The model under review builds one solid part; all positions refer to its coordinate system, in mm. A direction names the side the tool comes from. Round coordinates to 2 decimals unless told otherwise and drop trailing zeros. Write each loop counter-clockwise with the first axis right and the second up, starting at its lowest first coordinate (ties: lowest second). Pieces come first, ordered by that corner, then holes. Notation, with made-up numbers: (35.5, -36.5) - (47.5, -36.5) arc R22 cw to (47.5, -3.5) - close; hole circle Ø11 at (79.5, 10.5). An arc over 180 degrees is marked (long way). Return JSON: item names as keys, results as strings.
from build123d import *

# Parameters (mm, degrees)
BOX002_W          = 1
BOX002_H          = 4.5
BOX002_DEPTH      = 5.75
ARRAY001_COUNT    = 2
BOX001_W          = 2
BOX001_H          = 4.5
BOX001_DEPTH      = 5.5
ARRAY_COUNT       = 2
CYLINDER003_R     = 0.45
CYLINDER003_DEPTH = 2
CYLINDER004_R     = 0.45
CYLINDER004_DEPTH = 2
CYLINDER005_R     = 0.45
CYLINDER005_DEPTH = 2
CYLINDER006_R     = 0.45
CYLINDER006_DEPTH = 2
CYLINDER007_R     = 0.45
CYLINDER007_DEPTH = 2
CYLINDER008_R     = 0.45
CYLINDER008_DEPTH = 2
CYLINDER009_R     = 0.45
CYLINDER009_DEPTH = 2
CYLINDER010_R     = 0.45
CYLINDER010_DEPTH = 2
CYLINDER002_R     = 7
CYLINDER002_DEPTH = 10
CYLINDER001_R     = 11.5
CYLINDER001_DEPTH = 2
BOX_W             = 15
BOX_H             = 15
BOX_DEPTH         = 2
CYLINDER_R        = 13
CYLINDER_DEPTH    = 4.5
CHAMFER_SIZE      = 0.7


with BuildPart() as array001:
    # Box002 → Box002 (new body)
    with BuildSketch(Plane(origin=(8, -2.25, 0.75), x_dir=(1, 0, 0), z_dir=(0, 0, 1))):
        with Locations((0.5, 2.25)):
            Rectangle(BOX002_W, BOX002_H)
    extrude(amount=BOX002_DEPTH)

    # Array001: Array001 ×2 about axis
    array001_axis = Axis((0, 0, 0), (0, 0, 1))


with BuildPart() as array001_1:
    add(array001.part)
    for i in range(1, ARRAY001_COUNT):
        add(array001.part.rotate(array001_axis, i * 360 / ARRAY001_COUNT))


with BuildPart() as array:
    # Box001 → Box001 (new body)
    with BuildSketch(Plane(origin=(7, -2.25, 2), x_dir=(1, 0, 0), z_dir=(0, 0, 1))):
        with Locations((1, 2.25)):
            Rectangle(BOX001_W, BOX001_H)
    extrude(amount=BOX001_DEPTH)

    # Array: Array ×2 about axis
    array_axis = Axis((0, 0, 0), (0, 0, 1))


with BuildPart() as array_1:
    add(array.part)
    for i in range(1, ARRAY_COUNT):
        add(array.part.rotate(array_axis, i * 360 / ARRAY_COUNT))


with BuildPart() as cilindro003:
    # Cylinder003 → Cylinder003 (new body)
    with BuildSketch(Plane(origin=(6, 7.5, 4), x_dir=(1, 0, 0), z_dir=(0, 0, 1))):
        Circle(CYLINDER003_R)
    extrude(amount=CYLINDER003_DEPTH)


with BuildPart() as cilindro004:
    # Cylinder004 → Cylinder004 (new body)
    with BuildSketch(Plane(origin=(-6, 7.5, 4), x_dir=(1, 0, 0), z_dir=(0, 0, 1))):
        Circle(CYLINDER004_R)
    extrude(amount=CYLINDER004_DEPTH)


with BuildPart() as cilindro005:
    # Cylinder005 → Cylinder005 (new body)
    with BuildSketch(Plane(origin=(6, -7.5, 4), x_dir=(1, 0, 0), z_dir=(0, 0, 1))):
        Circle(CYLINDER005_R)
    extrude(amount=CYLINDER005_DEPTH)


with BuildPart() as cilindro006:
    # Cylinder006 → Cylinder006 (new body)
    with BuildSketch(Plane(origin=(-6, -7.5, 4), x_dir=(1, 0, 0), z_dir=(0, 0, 1))):
        Circle(CYLINDER006_R)
    extrude(amount=CYLINDER006_DEPTH)


with BuildPart() as cilindro007:
    # Cylinder007 → Cylinder007 (new body)
    with BuildSketch(Plane(origin=(7.5, 6, 4), x_dir=(1, 0, 0), z_dir=(0, 0, 1))):
        Circle(CYLINDER007_R)
    extrude(amount=CYLINDER007_DEPTH)


with BuildPart() as cilindro008:
    # Cylinder008 → Cylinder008 (new body)
    with BuildSketch(Plane(origin=(-7.5, 6, 4), x_dir=(1, 0, 0), z_dir=(0, 0, 1))):
        Circle(CYLINDER008_R)
    extrude(amount=CYLINDER008_DEPTH)


with BuildPart() as cilindro009:
    # Cylinder009 → Cylinder009 (new body)
    with BuildSketch(Plane(origin=(7.5, -6, 4), x_dir=(1, 0, 0), z_dir=(0, 0, 1))):
        Circle(CYLINDER009_R)
    extrude(amount=CYLINDER009_DEPTH)


with BuildPart() as cilindro010:
    # Cylinder010 → Cylinder010 (new body)
    with BuildSketch(Plane(origin=(-7.5, -6, 4), x_dir=(1, 0, 0), z_dir=(0, 0, 1))):
        Circle(CYLINDER010_R)
    extrude(amount=CYLINDER010_DEPTH)


with BuildPart() as cilindro002:
    # Cylinder002 → Cylinder002 (new body)
    with BuildSketch(Plane.XY):
        Circle(CYLINDER002_R)
    extrude(amount=CYLINDER002_DEPTH)


with BuildPart() as cilindro001:
    # Cylinder001 → Cylinder001 (new body)
    with BuildSketch(Plane.XY):
        Circle(CYLINDER001_R)
    extrude(amount=CYLINDER001_DEPTH)


with BuildPart() as cubo:
    # Box → Box (new body)
    with BuildSketch(Plane(origin=(-7.5, -7.5, 4), x_dir=(1, 0, 0), z_dir=(0, 0, 1))):
        with Locations((7.5, 7.5)):
            Rectangle(BOX_W, BOX_H)
    extrude(amount=BOX_DEPTH)


with BuildPart() as chamfer_body:
    # Cylinder → Cylinder (new body)
    with BuildSketch(Plane.XY):
        Circle(CYLINDER_R)
    extrude(amount=CYLINDER_DEPTH)

    # Fusion: union Cubo
    add(cubo.part)

    # Cut: cut Cilindro001
    add(cilindro001.part, mode=Mode.SUBTRACT)

    # Cut001: cut Cilindro002
    add(cilindro002.part, mode=Mode.SUBTRACT)

    # Fusion001: union Cilindro003, Cilindro004, Cilindro005, Cilindro006, Cilindro007, Cilindro008, Cilindro009, Cilindro010
    add(cilindro003.part)
    add(cilindro004.part)
    add(cilindro005.part)
    add(cilindro006.part)
    add(cilindro007.part)
    add(cilindro008.part)
    add(cilindro009.part)
    add(cilindro010.part)

    # Fusion002: union Array
    add(array_1.part)

    # Cut002: cut Array001
    add(array001_1.part, mode=Mode.SUBTRACT)

    # Chamfer
    chamfer_edges = [chamfer_body.edges().sort_by_distance(p)[0] for p in [
        (9, 0, 7.5),
        (-9, 0, 7.5),
    ]]
    chamfer(chamfer_edges, length=CHAMFER_SIZE)


solid = chamfer_body.part
(1) Wall thickness on line 1 (Y direction, x = 0, z = 4.3); line 2 (Y direction, x = 0, z = 1.3); line 3 (X direction, y = -2, z = 3.25): over which ranges is each line inside the solid? List them lowest first.
Filled in:
{"line 1": "y = -13 to -7, 7 to 13", "line 2": "y = -13 to -11.5, 11.5 to 13", "line 3": "x = -12.85 to -9, -8 to -6.71, 6.71 to 8, 9 to 12.85"}
(2) Add section B-B (y = 3.75). Write out the cut boundary in (x, z).
Filled in:
{"outline": "(-12.45, 0) - (-10.87, 0) - (-10.87, 2) - (-5.91, 2) - (-5.91, 6) - (-7.5, 6) - (-7.5, 4.5) - (-12.45, 4.5) - close; (5.91, 2) - (10.87, 2) - (10.87, 0) - (12.45, 0) - (12.45, 4.5) - (7.5, 4.5) - (7.5, 6) - (5.91, 6) - close"}
(3) Mouldability with a two-part tool opening along X and no side actions: class faces 6 (the flat face through (8, 0, 4)), 7 (the flat face through (7.8, -2.25, 6.3)), 8 (the cylindrical face through (7.95, -6.01, 5.24)) as released by +X, released by -X, zero draft, split by the parting line, or undercut.
Filled in:
{"face 6": "undercut", "face 7": "zero draft", "face 8": "released by +X"}
(4) For faces 1 (the flat face through (-7.5, -7, 5)), 2 (the flat face through (8.5, -2.25, 3.2)), 3 (the cylindrical face through (-6.01, -7.95, 5.24)), 4 (the flat face through (8.5, 0, 6.5)), 5 (the flat face through (-7, 0, 7)), list the 3-axis set-ups (+Z, -Z, +X, -X, +Y, -Y) from which the entire face can be reached by the end or side of a thin tool; tool diameter is ignored.
Filled in:
{"face 1": "+Z, -X, -Y", "face 2": "-Z", "face 3": "+Z, -Y", "face 4": "-Z, +X, +Y, -Y", "face 5": "+Z, +Y, -Y"}
(5) Add section A-A (x = 0). Write out the cut boundary in (y, z).
Filled in:
{"outline": "(-13, 0) - (-11.5, 0) - (-11.5, 2) - (-7, 2) - (-7, 6) - (-7.5, 6) - (-7.5, 4.5) - (-13, 4.5) - close; (7, 2) - (11.5, 2) - (11.5, 0) - (13, 0) - (13, 4.5) - (7.5, 4.5) - (7.5, 6) - (7, 6) - close"}
(6) Add section D-D (z = 3). Write out the cut boundary in (x, y), plus the area to 3 significant figures.
Filled in:
{"outline": "circle Ø26 at (0, 0); hole (-9, -2.25) - (-8, -2.25) - (-8, 2.25) - (-9, 2.25) - close; hole circle Ø14 at (0, 0); hole (8, -2.25) - (9, -2.25) - (9, 2.25) - (8, 2.25) - close", "area": "368 mm2"}
(7) Clearance check with flat-ended pins moving along their axes: pin 1 Ø1.6 at (x, z) = (-7.5, 5.5) entering from -Y; pin 2 Ø1.5 at (x, z) = (3, 4.5) entering from +Y; pin 3 Ø1 at (x, z) = (10, 4.5) entering from +Y. State where each tip first meets the part, or that it passes through.
Filled in:
{"pin 1": "stops at y = -7.5", "pin 2": "stops at y = 12.8", "pin 3": "stops at y = 8.87"}
